from build123d import *

# Parameters (mm, degrees)
SKETCH1_W           = 14.4
SKETCH1_H           = 14.4
BOSS_EXTRUDE1_DEPTH = 7.2
SKETCH2_R           = 2.415
BOSS_EXTRUDE2_DEPTH = 11.755
SKETCH3_R           = 2.415
BOSS_EXTRUDE3_DEPTH = 11.755
FILLET2_R           = 1


with BuildPart() as part:
    # Sketch1 → Boss-Extrude1 (new body, symmetric)
    with BuildSketch(Plane(origin=(0, 0, 0), x_dir=(1, 0, 0), z_dir=(0, 1, 0))):
        Rectangle(SKETCH1_W, SKETCH1_H)
    extrude(amount=BOSS_EXTRUDE1_DEPTH, both=True)

    # Sketch2 → Boss-Extrude2 (add, symmetric)
    with BuildSketch(Plane(origin=(0, 0, 0), x_dir=(0, 0, -1), z_dir=(1, 0, 0))):
        Circle(SKETCH2_R)
    extrude(amount=BOSS_EXTRUDE2_DEPTH, both=True)

    # Sketch3 → Boss-Extrude3 (add, symmetric)
    with BuildSketch(Plane(origin=(0, 0, 0), x_dir=(1, 0, 0), z_dir=(0, 1, 0))):
        Circle(SKETCH3_R)
    extrude(amount=BOSS_EXTRUDE3_DEPTH, both=True)

    # Fillet2
    fillet2_edges = [part.edges().sort_by_distance(p)[0] for p in [
        (-7.2, 7.2, 0),
        (0, 7.2, 7.2),
        (7.2, 7.2, 0),
        (0, -7.2, 7.2),
        (-7.2, -7.2, 0),
        (0, -7.2, -7.2),
        (7.2, -7.2, 0),
        (0, 7.2, -7.2),
        (7.2, 0, 7.2),
        (-7.2, 0, 7.2),
        (-7.2, 0, -7.2),
        (7.2, 0, -7.2),
    ]]
    fillet(fillet2_edges, radius=FILLET2_R)


solid = part.part
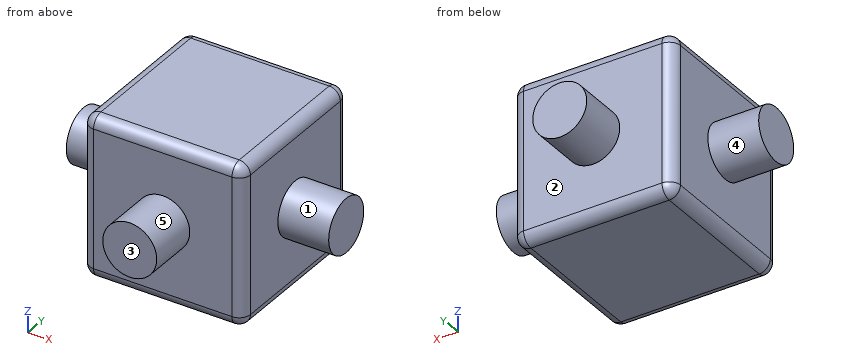
Work out the finished part from the listing and answer in its coordinate system (mm). Face numbers are marked on the shaded views. A direction names the side the tool comes from. Give positions to 0.01 mm unless a question says otherwise; leave off trailing zeros. Loops run counter-clockwise (first coordinate to the right, second up) from the corner with the lowest first, then second, coordinate; pieces in that order, holes last. Notation, with made-up numbers: (16.25, -15.75) - (71.25, -15.75) arc R30 cw to (71.25, 18.25) - close; hole circle Ø10 at (59, 63). An arc over 180 degrees is marked (long way). Answer in a Markdown table with one row per item. Add a question column.
Q1. The part is cut by section A-A (y = 0). Determine the outline of the cut face in (x, z) (3 decimals), and give its area (3 significant figures).
Q2. Consider line 1 along X through (y, z) = (-6.25, 0); line 2 along Z through (x, y) = (1, -8.5). Determine where each line is inside the solid, lowest interval first.
Q3. The part is cut by section C-C (z = 0). Determine the outline of the cut face in (x, y) (3 decimals).
Q4. A tool of negligible diameter and unlimited length cuts with its end or side. For the marked faces 1, 2, 3, 4 and 5, from which of +Z, -Z, +X, -X, +Y, -Y can it reach the whole face along a straight path? Write none if from no direction.
Q5. Each of these flat-tipped pins is pushed along its axis until it touches: P1, Ø3, axis at x = -4.5, z = -5.5, coming from the -Y side; P2, Ø1.5, axis at x = 1, z = 5, coming from the +Y side; P3, Ø1, axis at x = -1.5, y = 7.5, coming from the +Z side. Where does it stop, or does it pass through?
Q6. The part is cut by section B-B (x = -4). Determine the outline of the cut face in (y, z), and give its area (3 significant figures).
Solution:
| question | item | result |
|---|---|---|
| 1 | outline | (-11.755, -2.415) - (-7.2, -2.415) - (-7.2, -6.2) arc R1 ccw to (-6.2, -7.2) - (6.2, -7.2) arc R1 ccw to (7.2, -6.2) - (7.2, -2.415) - (11.755, -2.415) - (11.755, 2.415) - (7.2, 2.415) - (7.2, 6.2) arc R1 ccw to (6.2, 7.2) - (-6.2, 7.2) arc R1 ccw to (-7.2, 6.2) - (-7.2, 2.415) - (-11.755, 2.415) - close |
| 1 | area | 251 mm² |
| 2 | line 1 | x = -7.2 to 7.2 |
| 2 | line 2 | z = -2.2 to 2.2 |
| 3 | outline | (-11.755, -2.415) - (-7.2, -2.415) - (-7.2, -6.2) arc R1 ccw to (-6.2, -7.2) - (-2.415, -7.2) - (-2.415, -11.755) - (2.415, -11.755) - (2.415, -7.2) - (6.2, -7.2) arc R1 ccw to (7.2, -6.2) - (7.2, -2.415) - (11.755, -2.415) - (11.755, 2.415) - (7.2, 2.415) - (7.2, 6.2) arc R1 ccw to (6.2, 7.2) - (2.415, 7.2) - (2.415, 11.755) - (-2.415, 11.755) - (-2.415, 7.2) - (-6.2, 7.2) arc R1 ccw to (-7.2, 6.2) - (-7.2, 2.415) - (-11.755, 2.415) - close |
| 4 | face 1 | +X |
| 4 | face 2 | +Y |
| 4 | face 3 | +Z, -Z, +X, -X, -Y |
| 4 | face 4 | -X |
| 4 | face 5 | -Y |
| 5 | P1 | stops at y = -7.2 |
| 5 | P2 | stops at y = 7.2 |
| 5 | P3 | stops at z = 6.8 |
| 6 | outline | (-7.2, -6.2) arc R1 ccw to (-6.2, -7.2) - (6.2, -7.2) arc R1 ccw to (7.2, -6.2) - (7.2, 6.2) arc R1 ccw to (6.2, 7.2) - (-6.2, 7.2) arc R1 ccw to (-7.2, 6.2) - close |
| 6 | area | 207 mm² |
